Could you check a few things on this model? Use its own coordinates, in mm. Face numbers are marked on the shaded views. A direction names the side the tool comes from. Give positions to 0.01 mm unless a question says otherwise; leave off trailing zeros. Loops run counter-clockwise (first coordinate to the right, second up) from the corner with the lowest first, then second, coordinate; pieces in that order, holes last. Notation, with made-up numbers: M 48.25,-21.75 L 101.25,-21.75 A12 ccw 101.25,-17.75 Z; hole C -17.5,10 d2. An arc over 180 degrees is marked long. Use CSV: the item, a comma, the result in double quotes.
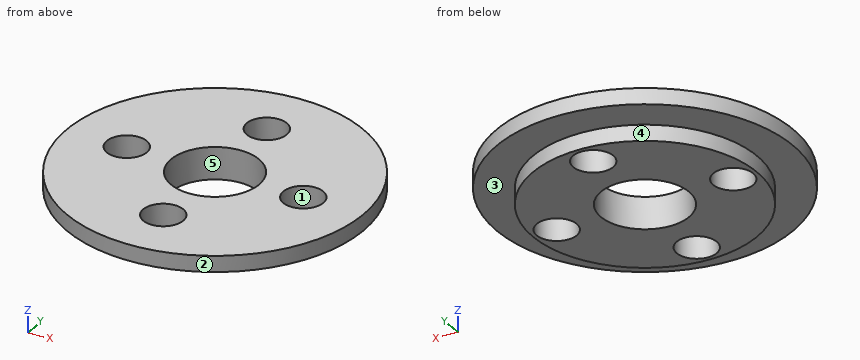
Autodesk Inventor part; units mm, degrees
ref_plane "YZ Plane" through (0, 0, 0) normal (1, 0, 0) x (0, 1, 0)
ref_plane "XZ Plane" through (0, 0, 0) normal (0, 1, 0) x (-1, 0, 0)
ref_plane "XY Plane" through (0, 0, 0) normal (0, 0, 1) x (1, 0, 0)
sketch "Sketch1" plane through (0, 0, 0) normal (0, 0, 1) x (1, 0, 0)
  circle A0 centre (0, 0) radius 14
  circle A1 centre (0, 0) radius 18.5
  line L0 (0, 0) -> (11, 0) construction
  dimension "d0" = 28
  dimension "d1" = 37
  dimension "d6" = 11
extrude "Extrusion1" add sketch "Sketch1" against normal blind 2 contours A0 | A1
extrude "Extrusion2" add sketch "Sketch1" against normal blind 4 contours A0
hole "Hole1" at (11, 0, 0) direction (0, 0, -1) diameter 5 end through all
pattern_circular "Circular Pattern1" count 4 over 360 about axis through (0, 0, -10) along (0, 0, 1) of "Hole1"
hole "Hole2" at (0, 0, 0) direction (0, 0, -1) diameter 11 end through all
properties part number "arm_coupler2" material "ABS Plastic"
1. If we mould it in two halves opening along X, with no side actions, what happens to the marked faces 1, 2 and 3? For each: +X half, -X half, draft (parallel to the pull), parting line (faces both ways), or undercut.
Outcome:
face 1,"undercut"
face 2,"parting line"
face 3,"draft"
2. I want a section at C-C, the plane z = -2.45. List the corners of the cut face in (x, y) for me, then the cut area to 3 significant figures.
Outcome:
outline,"C 0,0 d28; hole C -11,0 d5; hole C 0,0 d11; hole C 0,-11 d5; hole C 0,11 d5; hole C 11,0 d5"
area,"442 mm2"
3. I want a section at D-D, the plane y = 9.5. List the corners of the cut face in (x, z) for me, then the cut area to 3 significant figures.
Outcome:
outline,"M -15.87,-2 L -10.28,-2 L -10.28,-4 L -2,-4 L -2,0 L -15.87,0 Z; M 2,-4 L 10.28,-4 L 10.28,-2 L 15.87,-2 L 15.87,0 L 2,0 Z"
area,"88.6 mm2"
4. I want a section at A-A, the plane x = 0. List the corners of the cut face in (y, z) for me.
Outcome:
outline,"M -18.5,-2 L -14,-2 L -14,-4 L -13.5,-4 L -13.5,0 L -18.5,0 Z; M -8.5,-4 L -5.5,-4 L -5.5,0 L -8.5,0 Z; M 5.5,-4 L 8.5,-4 L 8.5,0 L 5.5,0 Z; M 13.5,-4 L 14,-4 L 14,-2 L 18.5,-2 L 18.5,0 L 13.5,0 Z"
5. Which directions (+Z, -Z, +X, -X, +Y, -Y) give clear straight access to the entire face, cutting with the end or side of a thin tool? Please do the marked faces 4 and 5.
Outcome:
face 4,"-Z"
face 5,"+Z, -Z"
6. I'm going to push flat-ended pins straight in: pin 1 Ø4 at (x, y) = (0, 11) entering from -Z; pin 2 Ø1.5 at (y, z) = (4, -1.5) entering from -X. Where does each tip first touch, or does it pass through?
Outcome:
pin 1,"through"
pin 2,"x = -18.21"
7. Please list where these lines run through material, in increasing order: line 1 (Y direction, x = 0, z = -1); line 2 (Y direction, x = 0, z = -3.15); line 3 (X direction, y = -2, z = -0.4).
Outcome:
line 1,"-18.5 to -13.5, -8.5 to -5.5, 5.5 to 8.5, 13.5 to 18.5"
line 2,"-14 to -13.5, -8.5 to -5.5, 5.5 to 8.5, 13.5 to 14"
line 3,"-18.39 to -12.5, -9.5 to -5.12, 5.12 to 9.5, 12.5 to 18.39"
